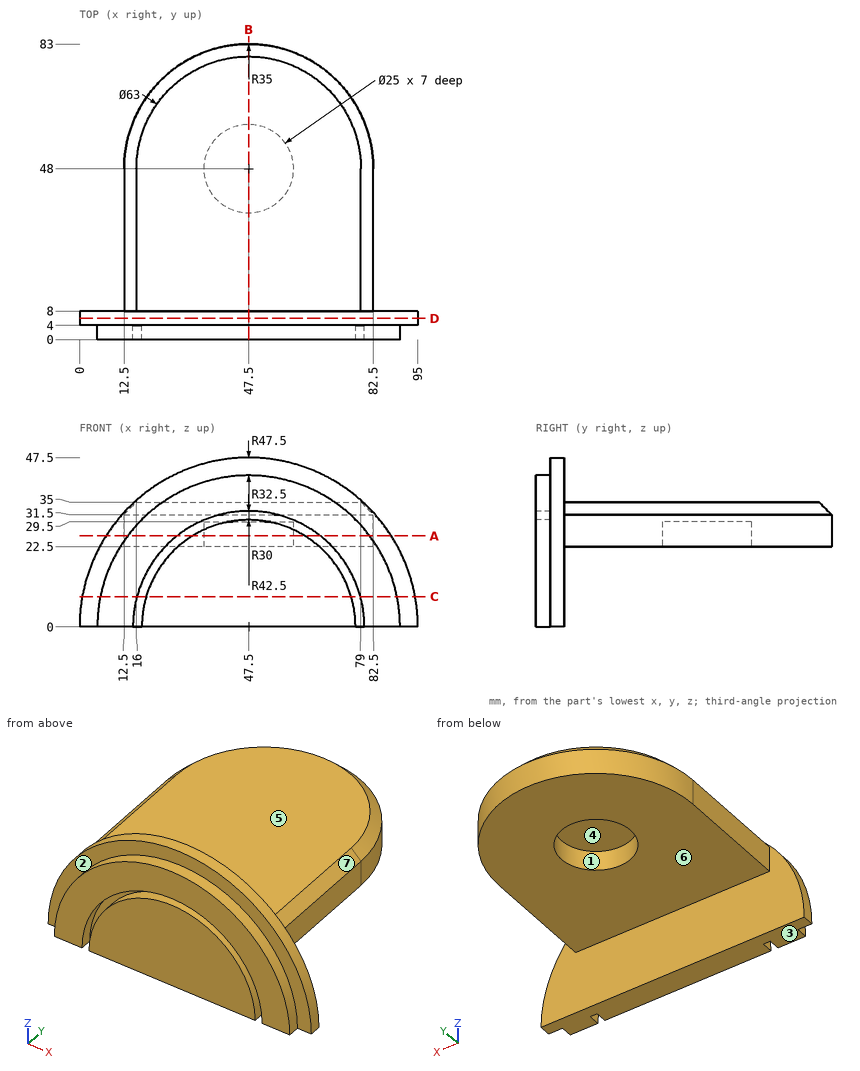
Drawing for the job (mm, zero at the part's lowest x, y, z). A direction names the side the tool comes from. Round coordinates to 2 decimals unless told otherwise and drop trailing zeros. Order: outer loops, then holes, each group sorted by start corner. A loop starts at its lowest first (then second) coordinate and runs counter-clockwise, first axis right, second up. Notation, with made-up numbers: (-0.5, -37) -> (9.5, -37) arc R26 ccw to (9.5, -16) -> close; hole circle Ø6 at (-27, 25). An arc over 180 degrees is marked (long way). Put each result on its own line as item: value.
Q1. Band-saw the part on A-A (z = 25.5). Give the cut face in (x, y).
From the geometry:
outline: (7.43, 4) -> (13.5, 4) -> (13.5, 0) -> (27.35, 0) -> (27.35, 4) -> (31.7, 4) -> (31.7, 0) -> (63.3, 0) -> (63.3, 4) -> (67.65, 4) -> (67.65, 0) -> (81.5, 0) -> (81.5, 4) -> (87.57, 4) -> (87.57, 8) -> (82.5, 8) -> (82.5, 48) arc R35 ccw to (12.5, 48) -> (12.5, 8) -> (7.43, 8) -> close; hole circle Ø25 at (47.5, 48)
Q2. Pin check, flat tips, straight feed: pin 1 Ø15 at (x, y) = (47.5, 48) entering from +Z; pin 2 Ø4.5 at (y, z) = (34, 25.5) entering from -X; pin 3 Ø6 at (y, z) = (49, 33.5) entering from +X; pin 4 Ø16 at (x, z) = (56, 12) entering from -Y. Stop position of each tip, or through.
From the geometry:
pin 1: stops at z = 35
pin 2: stops at x = 12.5
pin 3: stops at x = 82.5
pin 4: stops at y = 0
Q3. Band-saw the part on C-C (z = 8.5). Give the cut face in (x, y), and give its area (3 significant figures).
From the geometry:
outline: (0.77, 4) -> (5.86, 4) -> (5.86, 0) -> (16.13, 0) -> (16.13, 4) -> (18.73, 4) -> (18.73, 0) -> (76.27, 0) -> (76.27, 4) -> (78.87, 4) -> (78.87, 0) -> (89.14, 0) -> (89.14, 4) -> (94.23, 4) -> (94.23, 8) -> (0.77, 8) -> close
area: 686 mm2
Q4. Tool access for the marked faces 4, 5, 6 and 7: list every direction of +Z, -Z, +X, -X, +Y, -Y with a clear straight run to the whole face (end or side of a thin tool).
From the geometry:
face 4: -Z
face 5: +Z, +X, -X, +Y
face 6: -Z, +X, -X, +Y
face 7: +Z, +X, +Y
Q5. Band-saw the part on D-D (y = 6). Give the cut face in (x, z).
From the geometry:
outline: (0, 0) -> (95, 0) arc R47.5 ccw to start
Q6. Band-saw the part on B-B (x = 47.5). Give the cut face in (y, z).
From the geometry:
outline: (0, 0) -> (8, 0) -> (8, 22.5) -> (35.5, 22.5) -> (35.5, 29.5) -> (60.5, 29.5) -> (60.5, 22.5) -> (83, 22.5) -> (83, 31.5) -> (79.5, 35) -> (8, 35) -> (8, 47.5) -> (4, 47.5) -> (4, 42.5) -> (0, 42.5) -> (0, 32.5) -> (4, 32.5) -> (4, 30) -> (0, 30) -> close
Q7. Pull direction Y, two halves, no side cores. Call the marked faces 1, 2 and 3: pulls with the +Y half, pulls with the -Y half, needs draft (parallel to the pull), parting line crosses it, or undercut.
From the geometry:
face 1: undercut
face 2: pulls with the -Y half
face 3: needs draft
Q8. Wall check: line 1 (Y direction, x = 47, z = 28); line 2 (Z direction, x = 41.5, y = 40); line 3 (Y direction, x = 64.5, z = 18). Give the ranges that are in metal, low to high. Write a range as [from, to].
From the geometry:
line 1: y = [0, 35.51], [60.49, 83]
line 2: z = [29.5, 35]
line 3: y = [0, 8]
